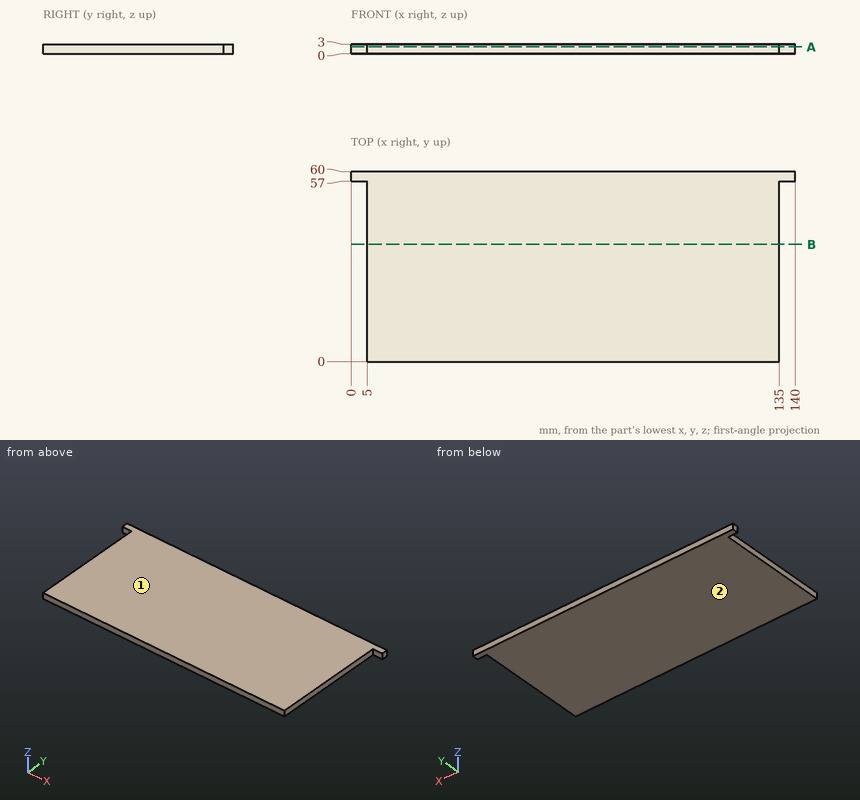
For this review, use the dimensioned drawing (mm, ordinates from the lowest corner) and the shaded views. Coordinates: 2 decimals unless noted, no trailing zeros. Write each loop counter-clockwise with the first axis right and the second up, starting at its lowest first coordinate (ties: lowest second). Pieces come first, ordered by that corner, then holes. Notation, with made-up numbers: (-5, 80) -> (17, 80) arc R24 ccw to (17, 99) -> close; hole circle Ø5 at (55, 73.25). An arc over 180 degrees is marked (long way). Put each result on its own line as item: value.
Q1. Wall thickness on L1, parallel to X at y = 38.5, z = 0.45: over which ranges is the line inside the solid? List them lowest first.
From the geometry:
L1: x = 5 to 135
Q2. The part is to be moulded in two halves that separate along Z. For the marked faces 1 and 2, say which applies: +Z half, -Z half, draft (parallel to the pull), parting line (faces both ways), or undercut.
From the geometry:
face 1: +Z half
face 2: -Z half
Q3. Take a section at A-A, the plane z = 2.1. State the section outline as (x, y) points, then the cut area to 3 significant figures.
From the geometry:
outline: (0, 57) -> (5, 57) -> (5, 0) -> (135, 0) -> (135, 57) -> (140, 57) -> (140, 60) -> (0, 60) -> close
area: 7,830 mm2
Q4. Clearance check with flat-ended pins moving along their axes: pin 1 Ø1.5 at (x, z) = (138, 2) entering from -Y; pin 2 Ø0.9 at (y, z) = (17, 1) entering from -X; pin 3 Ø1.5 at (y, z) = (15.5, 2) entering from +X. State where each tip first meets the part, or that it passes through.
From the geometry:
pin 1: stops at y = 57
pin 2: stops at x = 5
pin 3: stops at x = 135
Q5. Take a section at B-B, the plane y = 37. State the section outline as (x, z) points, then the cut area to 3 significant figures.
From the geometry:
outline: (5, 0) -> (135, 0) -> (135, 3) -> (5, 3) -> close
area: 390 mm2
